```python
from build123d import *

# Parameters (mm, degrees)
SKETCH1_W           = 176
SKETCH1_H           = 88.8
BOSS_EXTRUDE1_DEPTH = 1
SKETCH2_R           = 14.25
BOSS_EXTRUDE2_DEPTH = 16.7
FILLET1_R           = 1
SKETCH3_W           = 17.7
SKETCH3_H           = 17.7
BOSS_EXTRUDE3_DEPTH = 1.8
FILLET2_R           = 1
FILLET3_R           = 7
SKETCH4_R           = 6.25
BOSS_EXTRUDE4_DEPTH = 3.4
SKETCH7_R           = 7.5
BOSS_EXTRUDE5_DEPTH = 3.4
BOSS_EXTRUDE5_TAPER = 30


with BuildPart() as part:
    # Sketch1 → Boss-Extrude1 (new body)
    with BuildSketch(Plane(origin=(0, 0, 0), x_dir=(1, 0, 0), z_dir=(0, 1, 0))):
        Rectangle(SKETCH1_W, SKETCH1_H)
    extrude(amount=BOSS_EXTRUDE1_DEPTH)

    # Sketch2 → Boss-Extrude2 (add)
    with BuildSketch(Plane(origin=(0, 1, 0), x_dir=(1, 0, 0), z_dir=(0, 1, 0))):
        with Locations(Location((-56.75, 24.15, 0), (0, 0, 90))):
            Circle(SKETCH2_R)
    extrude(amount=BOSS_EXTRUDE2_DEPTH)

    # Fillet1
    fillet1_edges = [part.edges().sort_by_distance(p)[0] for p in [
        (-56.75, 17.7, -9.9),
    ]]
    fillet(fillet1_edges, radius=FILLET1_R)

    # Sketch3 → Boss-Extrude3 (add)
    with BuildSketch(Plane(origin=(0, 1, 0), x_dir=(1, 0, 0), z_dir=(0, 1, 0))):
        with Locations((-56.15, -25.55)):
            Rectangle(SKETCH3_W, SKETCH3_H)
        with Locations((57.15, 28.25)):
            Rectangle(SKETCH3_W, SKETCH3_H)
        with Locations((57.15, 0.55)):
            Rectangle(SKETCH3_W, SKETCH3_H)
    extrude(amount=BOSS_EXTRUDE3_DEPTH)

    # Fillet2
    fillet2_edges = [part.edges().sort_by_distance(p)[0] for p in [
        (-47.3, 1.9, 34.4),
        (-47.3, 1.9, 16.7),
        (-65, 1.9, 16.7),
        (-65, 1.9, 34.4),
        (66, 1.9, -19.4),
        (66, 1.9, -37.1),
        (48.3, 1.9, -37.1),
        (48.3, 1.9, -19.4),
        (66, 1.9, 8.3),
        (66, 1.9, -9.4),
        (48.3, 1.9, -9.4),
        (48.3, 1.9, 8.3),
    ]]
    fillet(fillet2_edges, radius=FILLET2_R)

    # Fillet3
    fillet3_edges = [part.edges().sort_by_distance(p)[0] for p in [
        (88, 0.5, 44.4),
        (-88, 0.5, 44.4),
        (-88, 0.5, -44.4),
        (88, 0.5, -44.4),
    ]]
    fillet(fillet3_edges, radius=FILLET3_R)

    # Sketch4 → Boss-Extrude4 (add)
    with BuildSketch(Plane(origin=(0, 2.8, 0), x_dir=(1, 0, 0), z_dir=(0, 1, 0))):
        with Locations(Location((-56.15, -25.55, 0), (0, 0, 90))):
            Circle(SKETCH4_R)
        with Locations(Location((57.15, 28.25, 0), (0, 0, 90))):
            Circle(SKETCH4_R)
        with Locations(Location((57.15, 0.55, 0), (0, 0, 90))):
            Circle(SKETCH4_R)
    extrude(amount=BOSS_EXTRUDE4_DEPTH)

    # Sketch7 → Boss-Extrude5 (add)
    with BuildSketch(Plane(origin=(0, 1, 0), x_dir=(1, 0, 0), z_dir=(0, 1, 0))):
        with Locations((57.15, -25.8)):
            Circle(SKETCH7_R)
    extrude(amount=BOSS_EXTRUDE5_DEPTH, taper=BOSS_EXTRUDE5_TAPER)


solid = part.part
```
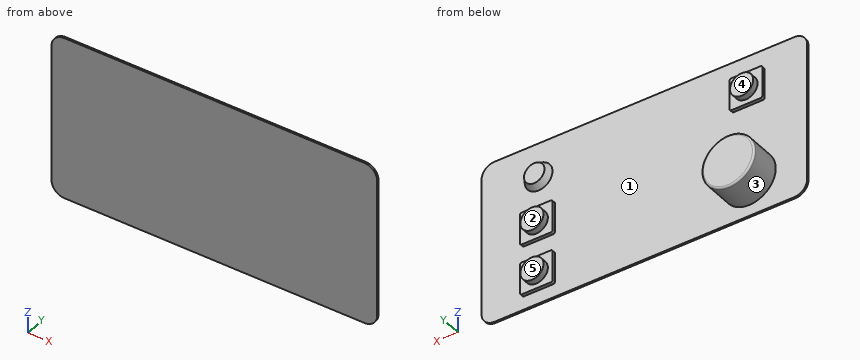
Check sheet for the modelled part. Datum: model origin and axes. Units: mm. Face numbers are marked on the shaded views. A direction names the side the tool comes from. Round coordinates to 2 decimals unless told otherwise and drop trailing zeros. Loops run counter-clockwise (first coordinate to the right, second up) from the corner with the lowest first, then second, coordinate; pieces in that order, holes last. Notation, with made-up numbers: (55.5, 73) - (88.5, 73) arc R7 ccw to (88.5, 80) - close; hole circle Ø4 at (27.25, 60.5). An arc over 180 degrees is marked (long way). Write item = value, one per line. Start each with the question number.
Q1. Access from +Z, -Z, +X, -X, +Y, -Y to the whole of each face (thin tool, end or side, straight path). Record for the marked faces 3, 4 and 5.
Q2. Section check D-D (x = -5.5). Record the boundary of the cut face in (y, z), plus the area to 3 significant figures.
Q3. Section check A-A (x = 57.15). Record the boundary of the cut face in (y, z), plus the area to 3 significant figures.
Q4. Section check C-C (y = 14.25). Record the boundary of the cut face in (x, z), plus the area to 3 significant figures.
Q5. Depth check by flat-ended pin: P1, Ø2, axis at x = 55, y = 1.5, coming from the +Z side; P2, Ø0.5, axis at y = 2, z = -28, coming from the -X side; P3, Ø12, axis at x = -15.5, z = -13, coming from the +Y side; P4, Ø8, axis at y = 15, z = -32.5, coming from the -X side. Enter the tip coordinate at first touch or a pass-through.
Q6. Section check B-B (z = -0.55). Record the boundary of the cut face in (x, y).
Q7. Thickness scan on L1, parallel to Y at x = 46, z = 28; L2, parallel to Y at x = 54, z = 7; L3, parallel to X at y = 3.25, z = 30. Record the ranges inside material, lowest first.
Q8. Release check for a two-part mould opening along X. For the marked faces 1 and 2 record: pulls with the +X half, pulls with the -X half, needs draft (parallel to the pull), parting line crosses it, or undercut.
Derived:
q1.face_3 = +Y
q1.face_4 = +Z, +X, -X, +Y
q1.face_5 = +Z, -Z, +X, +Y
q2.outline = (0, -44.4) - (1, -44.4) - (1, 44.4) - (0, 44.4) - close
q2.area = 88.8 mm^2
q3.outline = (0, -44.4) - (1, -44.4) - (1, -37.1) - (2.8, -37.1) - (2.8, -34.5) - (6.2, -34.5) - (6.2, -22) - (2.8, -22) - (2.8, -19.4) - (1, -19.4) - (1, -9.4) - (2.8, -9.4) - (2.8, -6.8) - (6.2, -6.8) - (6.2, 5.7) - (2.8, 5.7) - (2.8, 8.3) - (1, 8.3) - (1, 18.3) - (4.4, 20.26) - (4.4, 31.34) - (1, 33.3) - (1, 44.4) - (0, 44.4) - close
q3.area = 282 mm^2
q4.outline = circle Ø28.5 at (-56.75, -24.15)
q4.area = 638 mm^2
q5.P1 = 44.4
q5.P2 = -70.54
q5.P3 = 1
q5.P4 = -70.32
q6.outline = (-88, 0) - (88, 0) - (88, 1) - (66, 1) - (66, 2.8) - (63.4, 2.8) - (63.4, 6.2) - (50.9, 6.2) - (50.9, 2.8) - (48.3, 2.8) - (48.3, 1) - (-88, 1) - close
q7.L1 = 0 to 1
q7.L2 = 0 to 2.8
q7.L3 = -60.54 to -51.76, 52.59 to 61.71
q8.face_1 = undercut
q8.face_2 = needs draft
